Part model, mm, in its own coordinate system. Face numbers are marked on the shaded views. A direction names the side the tool comes from. Give positions to 0.01 mm unless a question says otherwise; leave off trailing zeros. Write each loop counter-clockwise with the first axis right and the second up, starting at its lowest first coordinate (ties: lowest second). Pieces come first, ordered by that corner, then holes. Notation, with made-up numbers: M 57,31 L 66,31 A17 ccw 66,51 Z; hole C 4,69.25 d6. An arc over 180 degrees is marked long. Answer as CSV lines item,"result". Start each with the question number.
Item 1: Band-saw the part on D-D, the plane z = 14.5. List the corners of the cut face in (x, y), then the cut area to 3 significant figures.
Item 2: Two-plate mould, pull along X, no slides. Class the marked faces 3, 4 and 5: +X half, -X half, draft (parallel to the pull), parting line (faces both ways), or undercut.
Item 3: Band-saw the part on A-A, the plane x = 0. List the corners of the cut face in (y, z).
Item 4: Pin check, flat tips, straight feed: pin 1 (1.7 mm diameter, centred on x = 0, y = -2, fed in from -Z); pin 2 (2 mm diameter, centred on x = 2, z = 13, fed in from -Y); pin 3 (1.6 mm diameter, centred on x = -1, z = 5.5, fed in from -Y). Stop position of each tip, or through.
Item 5: Wall check: L1, parallel to Z at x = -2.5, y = 1; L2, parallel to X at y = 1.5, z = 11.25; L3, parallel to Y at x = -2.75, z = 11. Give the ranges that are in metal, low to high. Write a range as from..to.
Item 6: 3-axis set-ups, long thin cutter, end or side, ignore diameter. For the marked faces 1 and 2: which of +Z, -Z, +X, -X, +Y, -Y reach the whole face in a straight line?
Item 7: Band-saw the part on C-C, the plane z = 10. List the corners of the cut face in (x, y), then the cut area to 3 significant figures.
Item 8: Band-saw the part on B-B, the plane y = 0. List the corners of the cut face in (x, z).
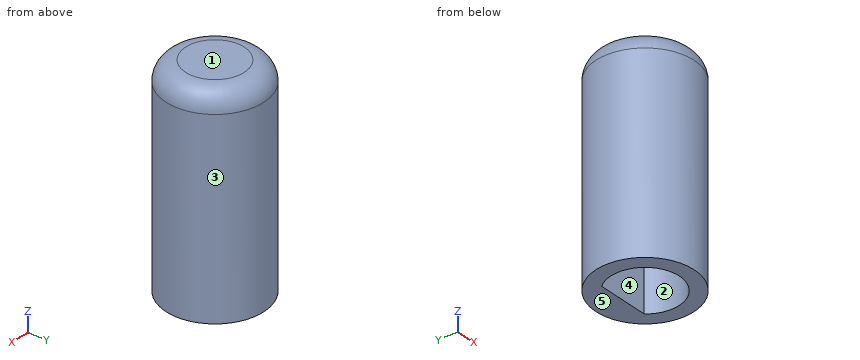
from build123d import *

# Parameters (mm, degrees)
SKETCH1_R           = 5
BOSS_EXTRUDE1_DEPTH = 11.5
SKETCH2_R           = 5
BOSS_EXTRUDE2_DEPTH = 10
FILLET2_R           = 2


with BuildPart() as part:
    # Sketch1 → Boss-Extrude1 (new body)
    with BuildSketch(Plane.XY):
        Circle(SKETCH1_R)
        with BuildLine():
            Line((-2.680951324, 2.25), (0, 2.25))
            Line((0, 2.25), (2.680951324, 2.25))
            ThreePointArc((2.680951324, 2.25), (0, -3.5), (-2.680951324, 2.25))
        make_face(mode=Mode.SUBTRACT)
    extrude(amount=BOSS_EXTRUDE1_DEPTH)

    # Sketch2 → Boss-Extrude2 (add)
    with BuildSketch(Plane.XY.offset(11.5)):
        Circle(SKETCH2_R)
    extrude(amount=BOSS_EXTRUDE2_DEPTH)

    # Fillet2
    fillet2_edges = [part.edges().sort_by_distance(p)[0] for p in [
        (-5, 0, 21.5),
    ]]
    fillet(fillet2_edges, radius=FILLET2_R)


solid = part.part
Output:
1,outline,"C 0,0 d10"
1,area,"78.5 mm²"
2,face 3,"parting line"
2,face 4,"undercut"
2,face 5,"draft"
3,outline,"M -5,0 L -3.5,0 L -3.5,11.5 L 2.25,11.5 L 2.25,0 L 5,0 L 5,19.5 A2 ccw 3,21.5 L -3,21.5 A2 ccw -5,19.5 Z"
4,pin 1,"z = 11.5"
4,pin 2,"y = -4.9"
4,pin 3,"y = -5"
5,L1,"11.5..21.5"
5,L2,"-4.77..-3.16, 3.16..4.77"
5,L3,"-4.18..-2.17, 2.17..4.18"
6,face 1,"+Z, +X, -X, +Y, -Y"
6,face 2,"-Z"
7,outline,"C 0,0 d10; hole M -2.68,2.25 A3.5 ccw long 2.68,2.25 Z"
7,area,"44.7 mm²"
8,outline,"M -5,0 L -3.5,0 L -3.5,11.5 L 3.5,11.5 L 3.5,0 L 5,0 L 5,19.5 A2 ccw 3,21.5 L -3,21.5 A2 ccw -5,19.5 Z"
